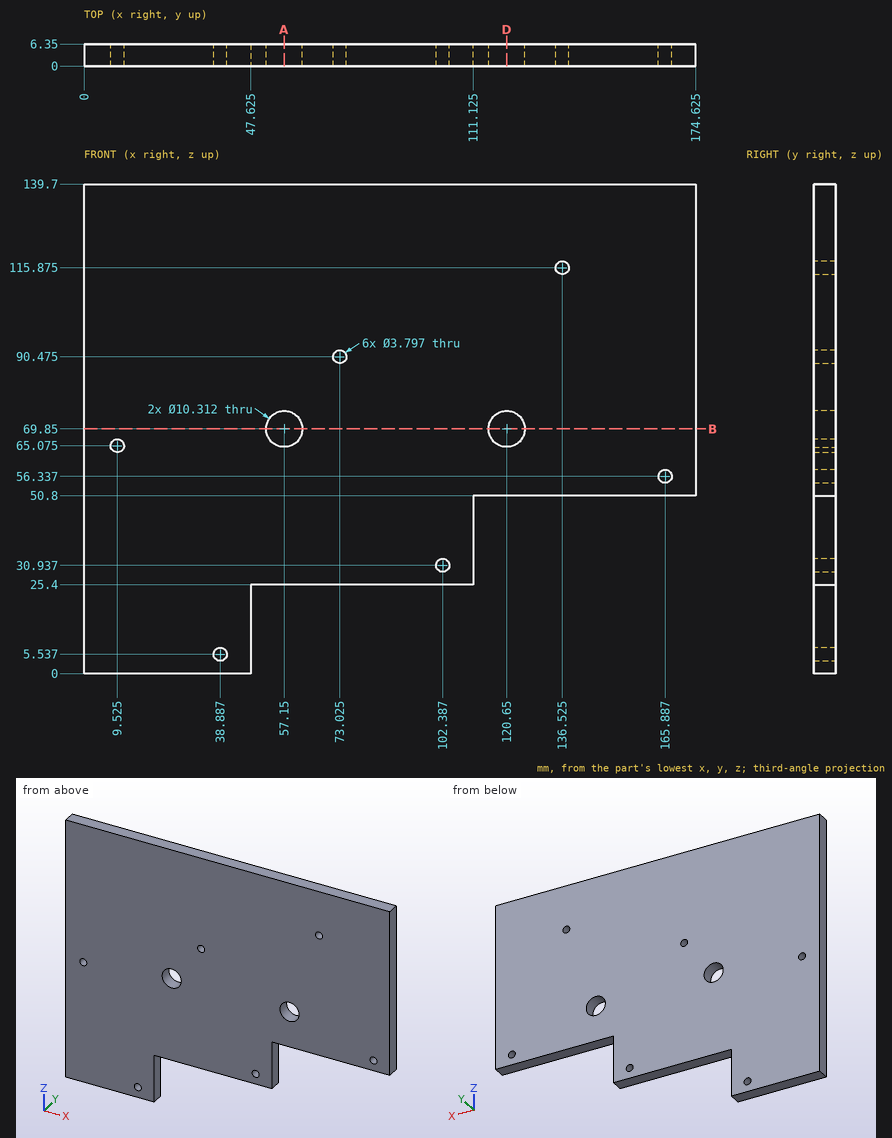
Check sheet for the drawn part. Datum: minimum x, y, z corner. Units: mm. Give positions to 0.01 mm unless a question says otherwise; leave off trailing zeros. Order: outer loops, then holes, each group sorted by start corner. A loop starts at its lowest first (then second) coordinate and runs counter-clockwise, first axis right, second up. Notation, with made-up numbers: (-14.75, -17.75) - (16.25, -17.75) arc R18 ccw to (16.25, -10.75) - close; hole circle Ø11 at (-33, 85). An arc over 180 degrees is marked (long way). Answer in a Markdown table with one row per item. Add a question column.
Q1. Gauge pin test, flat ends, axial feed: pin 1 (1.9 mm diameter, centred on y = 3.5, z = 7, fed in from +X) (3 decimals); pin 2 (3 mm diameter, centred on y = 2, z = 38, fed in from +X) (3 decimals); pin 3 (3 mm diameter, centred on x = 81, y = 4.5, fed in from -Z). Record the tip position at first contact, or that the pin passes through.
Q2. Cross-section at D-D, the plane x = 120.65. Enter the section's corners in (y, z), then the cut area to 3 significant figures.
Q3. Material ranges on probe 1 along X at (y, z) = (4.25, 69.85) (1 decimal); probe 2 along Z at (x, y) = (48.5, 5.25); probe 3 along X at (y, z) = (4.5, 45.5) (1 decimal), recorded low to high. Write a range as from..to.
Q4. Cross-section at A-A, the plane x = 57.15. Enter the section's corners in (y, z).
Q5. Cross-section at B-B, the plane z = 69.85. Count the separate pieces of the cut face and the enclosed holes in it, then the cut area to 3 significant figures.
Check values:
| question | item | result |
|---|---|---|
| 1 | pin 1 | stops at x = 47.625 |
| 1 | pin 2 | stops at x = 111.125 |
| 1 | pin 3 | stops at z = 25.4 |
| 2 | outline | (0, 50.8) - (6.35, 50.8) - (6.35, 64.69) - (0, 64.69) - close; (0, 75.01) - (6.35, 75.01) - (6.35, 139.7) - (0, 139.7) - close |
| 2 | area | 499 mm^2 |
| 3 | probe 1 | x = 0..52, 62.3..115.5, 125.8..174.6 |
| 3 | probe 2 | z = 25.4..139.7 |
| 3 | probe 3 | x = 0..111.1 |
| 4 | outline | (0, 25.4) - (6.35, 25.4) - (6.35, 64.69) - (0, 64.69) - close; (0, 75.01) - (6.35, 75.01) - (6.35, 139.7) - (0, 139.7) - close |
| 5 | separate pieces | 3 |
| 5 | enclosed holes | 0 |
| 5 | area | 978 mm^2 |
